from build123d import *

# Parameters (mm, degrees)
SKETCH3_W           = 19.05
SKETCH3_H           = 19.05
SKETCH3_W_2         = 16.5608
SKETCH3_H_2         = 16.5608
BOSS_EXTRUDE1_DEPTH = 254.635
FILLET1_R           = 1.2446
CUT_EXTRUDE1_REACH  = 257.524
SKETCH4_R           = 2.413
CUT_EXTRUDE3_START  = -19.05
CUT_EXTRUDE3_DEPTH  = 6.35
LPATTERN2_COUNT     = 8
LPATTERN2_PITCH     = 50.8


with BuildPart() as part:
    # Sketch3 → Boss-Extrude1 (new, symmetric)
    with BuildSketch(Plane.XY):
        Rectangle(SKETCH3_W, SKETCH3_H)
        Rectangle(SKETCH3_W_2, SKETCH3_H_2, mode=Mode.SUBTRACT)
    extrude(amount=BOSS_EXTRUDE1_DEPTH, both=True)

    # Fillet1
    fillet1_edges = [part.edges().sort_by_distance(p)[0] for p in [
        (-8.2804, -8.2804, 0),
        (8.2804, -8.2804, 0),
        (8.2804, 8.2804, 0),
        (-8.2804, 8.2804, 0),
        (9.525, -9.525, 0),
        (-9.525, -9.525, 0),
        (-9.525, 9.525, 0),
        (9.525, 9.525, 0),
    ]]
    fillet(fillet1_edges, radius=FILLET1_R)

    # Sketch4 → Cut-Extrude1 (cut, up to next)
    with BuildSketch(Plane(origin=(0, 9.525, 0), x_dir=(1, 0, 0), z_dir=(0, 1, 0)), mode=Mode.PRIVATE) as cut_extrude1_sk1:
        with Locations(Location((0, 159.385, 0), (0, 0, 270))):
            Circle(SKETCH4_R)
    cut_extrude1_tool1 = extrude(cut_extrude1_sk1.sketch, amount=-CUT_EXTRUDE1_REACH, mode=Mode.PRIVATE) & part.part
    # Sketch4 → Cut-Extrude1 (cut, up to next)
    with BuildSketch(Plane(origin=(0, 9.525, 0), x_dir=(1, 0, 0), z_dir=(0, 1, 0)), mode=Mode.PRIVATE) as cut_extrude1_sk2:
        with Locations(Location((0, 108.585, 0), (0, 0, 270))):
            Circle(SKETCH4_R)
    cut_extrude1_tool2 = extrude(cut_extrude1_sk2.sketch, amount=-CUT_EXTRUDE1_REACH, mode=Mode.PRIVATE) & part.part
    # Sketch4 → Cut-Extrude1 (cut, up to next)
    with BuildSketch(Plane(origin=(0, 9.525, 0), x_dir=(1, 0, 0), z_dir=(0, 1, 0)), mode=Mode.PRIVATE) as cut_extrude1_sk3:
        with Locations(Location((0, 57.785, 0), (0, 0, 270))):
            Circle(SKETCH4_R)
    cut_extrude1_tool3 = extrude(cut_extrude1_sk3.sketch, amount=-CUT_EXTRUDE1_REACH, mode=Mode.PRIVATE) & part.part
    # Sketch4 → Cut-Extrude1 (cut, up to next)
    with BuildSketch(Plane(origin=(0, 9.525, 0), x_dir=(1, 0, 0), z_dir=(0, 1, 0)), mode=Mode.PRIVATE) as cut_extrude1_sk4:
        with Locations(Location((0, 6.985, 0), (0, 0, 270))):
            Circle(SKETCH4_R)
    cut_extrude1_tool4 = extrude(cut_extrude1_sk4.sketch, amount=-CUT_EXTRUDE1_REACH, mode=Mode.PRIVATE) & part.part
    # Sketch4 → Cut-Extrude1 (cut, up to next)
    with BuildSketch(Plane(origin=(0, 9.525, 0), x_dir=(1, 0, 0), z_dir=(0, 1, 0)), mode=Mode.PRIVATE) as cut_extrude1_sk5:
        with Locations(Location((0, -43.815, 0), (0, 0, 270))):
            Circle(SKETCH4_R)
    cut_extrude1_tool5 = extrude(cut_extrude1_sk5.sketch, amount=-CUT_EXTRUDE1_REACH, mode=Mode.PRIVATE) & part.part
    # Sketch4 → Cut-Extrude1 (cut, up to next)
    with BuildSketch(Plane(origin=(0, 9.525, 0), x_dir=(1, 0, 0), z_dir=(0, 1, 0)), mode=Mode.PRIVATE) as cut_extrude1_sk6:
        with Locations(Location((0, -94.615, 0), (0, 0, 270))):
            Circle(SKETCH4_R)
    cut_extrude1_tool6 = extrude(cut_extrude1_sk6.sketch, amount=-CUT_EXTRUDE1_REACH, mode=Mode.PRIVATE) & part.part
    # Sketch4 → Cut-Extrude1 (cut, up to next)
    with BuildSketch(Plane(origin=(0, 9.525, 0), x_dir=(1, 0, 0), z_dir=(0, 1, 0)), mode=Mode.PRIVATE) as cut_extrude1_sk7:
        with Locations(Location((0, -145.415, 0), (0, 0, 270))):
            Circle(SKETCH4_R)
    cut_extrude1_tool7 = extrude(cut_extrude1_sk7.sketch, amount=-CUT_EXTRUDE1_REACH, mode=Mode.PRIVATE) & part.part
    # Sketch4 → Cut-Extrude1 (cut, up to next)
    with BuildSketch(Plane(origin=(0, 9.525, 0), x_dir=(1, 0, 0), z_dir=(0, 1, 0)), mode=Mode.PRIVATE) as cut_extrude1_sk8:
        with Locations(Location((0, -196.215, 0), (0, 0, 270))):
            Circle(SKETCH4_R)
    cut_extrude1_tool8 = extrude(cut_extrude1_sk8.sketch, amount=-CUT_EXTRUDE1_REACH, mode=Mode.PRIVATE) & part.part
    add(cut_extrude1_tool1.solids().sort_by_distance((0, 9.525, -159.385))[0], mode=Mode.SUBTRACT)
    add(cut_extrude1_tool2.solids().sort_by_distance((0, 9.525, -108.585))[0], mode=Mode.SUBTRACT)
    add(cut_extrude1_tool3.solids().sort_by_distance((0, 9.525, -57.785))[0], mode=Mode.SUBTRACT)
    add(cut_extrude1_tool4.solids().sort_by_distance((0, 9.525, -6.985))[0], mode=Mode.SUBTRACT)
    add(cut_extrude1_tool5.solids().sort_by_distance((0, 9.525, 43.815))[0], mode=Mode.SUBTRACT)
    add(cut_extrude1_tool6.solids().sort_by_distance((0, 9.525, 94.615))[0], mode=Mode.SUBTRACT)
    add(cut_extrude1_tool7.solids().sort_by_distance((0, 9.525, 145.415))[0], mode=Mode.SUBTRACT)
    add(cut_extrude1_tool8.solids().sort_by_distance((0, 9.525, 196.215))[0], mode=Mode.SUBTRACT)

    # Sketch6 → Cut-Extrude3 (cut)
    with BuildSketch(Plane.ZY.offset(9.525).offset(CUT_EXTRUDE3_START)):
        Polygon((-182.118, -1.651), (-187.198, -1.651), (-187.198, 9.525), (-192.278, 9.525), (-192.278, -6.477), (-182.118, -6.477), (-177.292, -6.477), (-177.292, -1.651), align=None)
    cut_extrude3 = extrude(amount=CUT_EXTRUDE3_DEPTH, mode=Mode.SUBTRACT)

    # LPattern2: Cut-Extrude3 ×8
    with Locations(*[(0, 0, i * LPATTERN2_PITCH) for i in range(1, LPATTERN2_COUNT)]):
        add(cut_extrude3, mode=Mode.SUBTRACT)


solid = part.part
Verification items for the finished model (mm, model axes). A direction names the side the tool comes from. Round coordinates to 2 decimals unless told otherwise and drop trailing zeros. Loops run counter-clockwise (first coordinate to the right, second up) from the corner with the lowest first, then second, coordinate; pieces in that order, holes last. Notation, with made-up numbers: (-16, 61.5) - (37, 61.5) arc R15 ccw to (37, 75.5) - close; hole circle Ø9 at (28.25, 18.25). An arc over 180 degrees is marked (long way). Write item = value, one per line.
Q1. Material ranges on L1, parallel to Y at x = -6.5, z = 82 (3 decimals); L2, parallel to Y at x = -7.5, z = -36.5 (3 decimals), recorded low to high.
Here are the results:
L1 = -9.525 to -8.28, 8.28 to 9.525
L2 = -9.525 to -8.191, 8.191 to 9.525
Q2. Mould release check, pull along Y, two halves, no side actions. Record for faces 1 (the flat face through (0, 9.525, 4)), 2 (the flat face through (-9, 0, 254.635)), 3 (the flat face through (0, -8.28, 4)): +Y half, -Y half, draft (parallel to the pull), parting line (faces both ways), or undercut.
Here are the results:
face_1 = +Y half
face_2 = draft
face_3 = undercut
Q3. Sectioned sample at A-A on z = 0. Record the boundary of the cut face in (x, y) (3 decimals).
Here are the results:
outline = (-9.525, -8.28) arc R1.245 ccw to (-8.28, -9.525) - (8.28, -9.525) arc R1.245 ccw to (9.525, -8.28) - (9.525, 8.28) arc R1.245 ccw to (8.28, 9.525) - (-8.28, 9.525) arc R1.245 ccw to (-9.525, 8.28) - close; hole (-8.28, -7.036) arc R1.245 ccw to (-7.036, -8.28) - (7.036, -8.28) arc R1.245 ccw to (8.28, -7.036) - (8.28, 7.036) arc R1.245 ccw to (7.036, 8.28) - (-7.036, 8.28) arc R1.245 ccw to (-8.28, 7.036) - close
Q4. Depth check by flat-ended pin: pin 1 (1 mm diameter, centred on x = 9, z = -29.5, fed in from +Y); pin 2 (1.4 mm diameter, centred on x = 8.5, z = 124.5, fed in from -Y) (3 decimals); pin 3 (1 mm diameter, centred on x = 9, z = 116.5, fed in from +Y); pin 4 (1.9 mm diameter, centred on x = 7, y = 6, fed in from -Z). Enter the tip coordinate at first touch or a pass-through.
Here are the results:
pin_1 = 9.51
pin_2 = -9.525
pin_3 = -6.48
pin_4 = through
Q5. Tool access check on faces 4 (the flat face through (8.28, 0, 4)), 5 (the flat face through (-9.525, 0, 4)). Record the directions out of +Z, -Z, +X, -X, +Y, -Y that give a thin tool (end or side, any length) a straight path to the whole face; none if there is none.
Here are the results:
face_4 = +Z, -Z
face_5 = +Z, -Z, -X, +Y, -Y
